from build123d import *

# Parameters (mm, degrees)
F2_R     = 2.4
F3_DEPTH = 25


with BuildPart() as f1:
    # F0 (on Top) → F1 (revolve)
    with BuildSketch(Plane.XY):
        Polygon((-29.93912, 22.017142), (-31.93912, 22.017142), (-31.93912, 19.824239), (-31.93912, 18.824239), (-21.077308, 18.824239), (-21.077308, 21.274239), (-22.577308, 21.274239), (-22.577308, 21.574239), (-29.93912, 22.717142), align=None)
    revolve(axis=Axis((-26.508214, 18.824239, 0), (-1, 0, 0)))

    # F2 (on face) → F3 (cut)
    with BuildSketch(Plane(origin=(-31.93912, 0, 0), x_dir=(0, -1, 0), z_dir=(-1, 0, 0))):
        with Locations((-18.824239, 0)):
            Circle(F2_R)
    extrude(amount=-F3_DEPTH, mode=Mode.SUBTRACT)


solid = f1.part
Model file for the job. Use its own axes, mm. Give positions to 0.01 mm unless a question says otherwise; leave off trailing zeros. Loops run counter-clockwise (first coordinate to the right, second up) from the corner with the lowest first, then second, coordinate; pieces in that order, holes last.
Item 1: Drop flat-ended pins along their axis: P1, Ø1.5, axis at x = -23, y = 21, coming from the +Z side; P2, Ø1, axis at x = -26, y = 17, coming from the -Z side; P3, Ø3, axis at x = -25, z = 2, coming from the +Y side. Give the stop position or say it passes through.
Check values:
P1: stops at z = 2.45
P2: stops at z = -3.02
P3: stops at y = 21.99
Item 2: Slice it at A-A (z = 0). Write the cut outline in (x, y).
Check values:
outline: (-31.94, 15.63) - (-29.94, 15.63) - (-29.94, 14.93) - (-22.58, 16.07) - (-22.58, 16.37) - (-21.08, 16.37) - (-21.08, 16.42) - (-31.94, 16.42) - close; (-31.94, 21.22) - (-21.08, 21.22) - (-21.08, 21.27) - (-22.58, 21.27) - (-22.58, 21.57) - (-29.94, 22.72) - (-29.94, 22.02) - (-31.94, 22.02) - close
Item 3: Drill centre lines: line 1 along Z through (x, y) = (-26, 19.75); line 2 along Z through (x, y) = (-23.5, 18); line 3 along X through (y, z) = (16.75, -1.5). Where is each one in solid material? Low to high.
Check values:
line 1: z = -3.15 to -2.21, 2.21 to 3.15
line 2: z = -2.77 to -2.25, 2.25 to 2.77
line 3: x = -31.94 to -22.58
Item 4: Slice it at C-C (x = -26.25). Write the cut outline in (y, z), plus the area to 3 significant figures.
Check values:
outline: circle Ø6.64 at (18.82, 0); hole circle Ø4.8 at (18.82, 0)
area: 16.5 mm2
Item 5: Mould opens along Z. For faces 1 (the face through (-25.49, 21.78, 1.23)), 2 (the face through (-31.939, 16, 0)), 3 (the face through (-26.58, 21.22, 0.11)) say: +Z half, -Z half, draft (parallel to the pull), parting line (faces both ways), or undercut.
Check values:
face 1: parting line
face 2: draft
face 3: undercut
Item 6: Slice it at B-B (x = -30.25). Write the cut outline in (y, z).
Check values:
outline: circle Ø6.39 at (18.82, 0); hole circle Ø4.8 at (18.82, 0)
